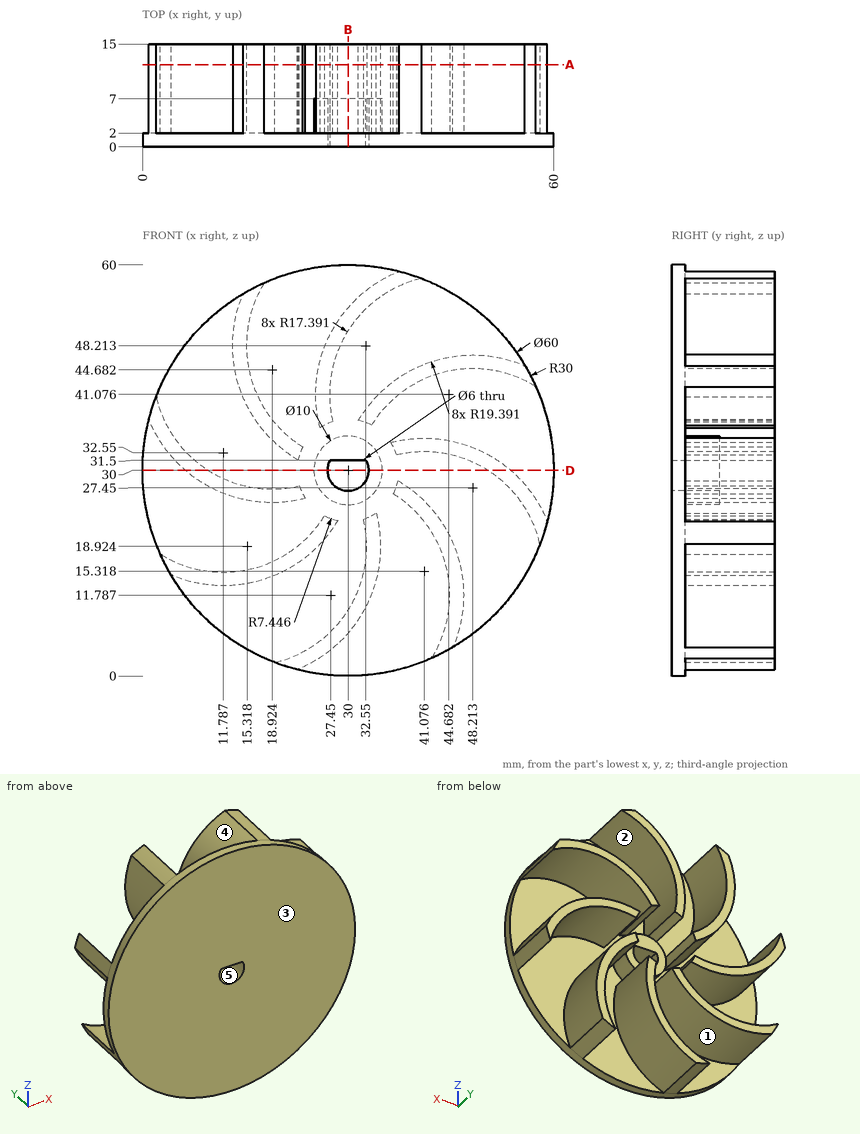
Study the drawing (mm; zero at the part's minimum x, y, z) and answer. A direction names the side the tool comes from. Round coordinates to 2 decimals unless told otherwise and drop trailing zeros. Write each loop counter-clockwise with the first axis right and the second up, starting at its lowest first coordinate (ties: lowest second). Pieces come first, ordered by that corner, then holes.
1) A cutting plane is placed at A-A on y = 12. Give the number of separate pieces and of enclosed holes in the cut face.
2) A cutting plane is placed at D-D on z = 30. Determine the outline of the cut face in (x, y).
3) Consider probe 1 along X at (y, z) = (5, 30) (1 decimal); probe 2 along Z at (x, y) = (30, 1.5); probe 3 along X at (y, z) = (8.75, 36.5) (1 decimal). Determine where each line is inside the solid, lowest interval first.
4) Determine the mould class of the marked faces 1, 2 and 3 for opening direction X: pulls with the +X half, pulls with the -X half, needs draft (parallel to the pull), parting line crosses it, or undercut.
5) Flat-ended cylindrical pins translate along their axes: P1, Ø1.5, axis at y = 12.5, z = 8, coming from the +X side; P2, Ø8, axis at x = 32, z = 28, coming from the +Y side; P3, Ø6, axis at y = 9.5, z = 24, coming from the +X side. Find the tip coordinate at first contact, or state that the pin passes through.
6) A cutting plane is placed at B-B on x = 30. Determine the outline of the cut face in (y, z).
7) Which of the six approach directions +Z, -Z, +X, -X, +Y, -Y give full straight-line access (tool end or side, diameter ignored) to the marked faces 4 and 5?
Entries:
1. separate pieces: 8
1. enclosed holes: 0
2. outline: (0, 0) - (27, 0) - (27, 7) - (25, 7) - (25, 2) - (9.6, 2) - (9.6, 15) - (6.26, 15) - (6.26, 2) - (0, 2) - close; (33, 0) - (60, 0) - (60, 2) - (53.74, 2) - (53.74, 15) - (50.4, 15) - (50.4, 2) - (35, 2) - (35, 7) - (33, 7) - close
3. probe 1: x = 6.3 to 9.6, 25 to 27, 33 to 35, 50.4 to 53.7
3. probe 2: z = 0 to 27, 31.5 to 60
3. probe 3: x = 1.3 to 3.6, 17.1 to 19.7, 25.8 to 26.4
4. face 1: undercut
4. face 2: undercut
4. face 3: needs draft
5. P1: stops at x = 46.6
5. P2: stops at y = 7
5. P3: stops at x = 59.06
6. outline: (0, 0) - (2, 0) - (2, 6.26) - (15, 6.26) - (15, 9.6) - (2, 9.6) - (2, 25) - (7, 25) - (7, 27) - (0, 27) - close; (0, 31.5) - (7, 31.5) - (7, 35) - (2, 35) - (2, 50.4) - (15, 50.4) - (15, 53.74) - (2, 53.74) - (2, 60) - (0, 60) - close
7. face 4: +Y
7. face 5: +Y, -Y
